from build123d import *

# Parameters (mm, degrees)
ESQUISSE1_W   = 1120
ESQUISSE1_H   = 147.955968354
ESQUISSE1_W_2 = 250
ESQUISSE1_H_2 = 75


with BuildPart() as part:
    # Esquisse1 → Révolution1 (revolve)
    with BuildSketch(Plane.XY, mode=Mode.PRIVATE) as r_volution1_sk:
        with Locations((473.529943231, -73.977984177)):
            Rectangle(ESQUISSE1_W, ESQUISSE1_H)
        with Locations((-241.470056769, -37.5)):
            Rectangle(ESQUISSE1_W_2, ESQUISSE1_H_2)
        Polygon((-86.470056769, -147.955968354), (-86.470056769, 0), (-116.470056769, 0), (-116.470056769, -75), (-116.470056769, -117.955968354), align=None)
        Polygon((1133.529943231, -247.955968354), (1133.529943231, 0), (1033.529943231, 0), (1033.529943231, -147.955968354), align=None)
        Polygon((1233.529943231, -300), (1233.529943231, 0), (1133.529943231, 0), (1133.529943231, -247.955968354), (1133.529943231, -400), align=None)
    revolve(r_volution1_sk.sketch.rotate(Axis((-576.0190019, 0, 0), (1, 0, 0)), 270), axis=Axis((-576.0190019, 0, 0), (1, 0, 0)))


solid = part.part
For this review, take the finished solid that the model builds, in its own axes (mm). A direction names the side the tool comes from. Round coordinates to 2 decimals unless told otherwise and drop trailing zeros. Write each loop counter-clockwise with the first axis right and the second up, starting at its lowest first coordinate (ties: lowest second). Pieces come first, ordered by that corner, then holes. Notation, with made-up numbers: (56, 34.25) -> (105, 34.25) arc R18 cw to (105, 66.25) -> close; hole circle Ø8 at (1, 33). An arc over 180 degrees is marked (long way). Put each result on its own line as item: value.
Q1. Clearance check with flat-ended pins moving along their axes: pin 1 Ø3 at (y, z) = (-80.5, -68.5) entering from -X; pin 2 Ø1.5 at (y, z) = (218.5, -175) entering from -X; pin 3 Ø3 at (y, z) = (83, 300) entering from +X. State where each tip first meets the part, or that it passes through.
Determined:
pin 1: stops at x = -116.47
pin 2: stops at x = 1133.53
pin 3: stops at x = 1223.76
Q2. Consider section C-C on x = 310. State the section outline as (y, z) points, and give its area (3 significant figures).
Determined:
outline: circle Ø295.91 at (0, 0)
area: 68,800 mm^2
Q3. To check wall thickness, follow L1, parallel to X at y = -159, z = 191; L2, parallel to X at y = -75, z = 27.5; L3, parallel to Y at x = 71.5, z = -116. State the ranges of each line that lie inside material, in increasing order. Write a range as [from, to].
Determined:
L1: x = [1133.53, 1233.53]
L2: x = [-116.47, 1233.53]
L3: y = [-91.84, 91.84]
Q4. Consider section D-D on x = 1053.5. State the section outline as (y, z) points.
Determined:
outline: circle Ø335.85 at (0, 0)
Q5. Consider section A-A on y = 0. State the section outline as (x, z) points, and give its area (3 significant figures).
Determined:
outline: (-366.47, -75) -> (-116.47, -75) -> (-116.47, -117.96) -> (-86.47, -147.96) -> (1033.53, -147.96) -> (1133.53, -247.96) -> (1133.53, -400) -> (1233.53, -300) -> (1233.53, 300) -> (1133.53, 400) -> (1133.53, 247.96) -> (1033.53, 147.96) -> (-86.47, 147.96) -> (-116.47, 117.96) -> (-116.47, 75) -> (-366.47, 75) -> close
area: 486,000 mm^2
Q6. Machinability: for faces 1 (the cylindrical face through (481.37, 90.03, -117.41)), 2 (the conical face through (1228.674, -302.261, -39.686)), which of the approach directions +Z, -Z, +X, -X, +Y, -Y give a long, thin tool a straight path to every point of the face, cutting with its end or side? Answer none if there is none.
Determined:
face 1: -X
face 2: +X
